from build123d import *

# Parameters (mm, degrees)
F0_W     = 5.842
F0_H     = 12.7
F0_R     = 3.175
F2_DEPTH = 25.4


with BuildPart() as f1:
    # F0 (on Front) → F1 (revolve)
    with BuildSketch(Plane.XZ):
        with Locations((2.921, 6.35)):
            Rectangle(F0_W, F0_H)
        Polygon((5.842, 12.7), (5.842, 0), (66.294, 0), (66.294, 12.7), (56.134, 12.7), (56.134, 10.16), (10.16, 10.16), (10.16, 12.7), align=None)
    revolve(axis=Axis((33.147, 0, 0), (-1, 0, 0)))

    # F0 (on Front) → F2 (join)
    with BuildSketch(Plane.XZ):
        with BuildLine():
            Line((-0.9398, 0), (0, 0))
            Line((0, 0), (0, 12.7))
            Line((0, 12.7), (5.842, 12.7))
            Line((5.842, 12.7), (5.842, 15.24))
            Line((5.842, 15.24), (-0.508, 15.24))
            Line((-0.508, 15.24), (-10.88063, 3.847543))
            ThreePointArc((-10.88063, 3.847543), (-4.591961, 5.329721), (-0.9398, 0))
        make_face()
        with BuildLine():
            ThreePointArc((-8.182663, -5.506983), (-3.195791, -4.549339), (-0.9398, 0))
            ThreePointArc((-0.9398, 0), (-4.591961, 5.329721), (-10.88063, 3.847543))
            ThreePointArc((-10.88063, 3.847543), (-12.145978, -1.583727), (-8.182663, -5.506983))
        make_face()
        with Locations((-6.6548, 0)):
            Circle(F0_R, mode=Mode.SUBTRACT)
        with BuildLine():
            Line((5.842, 0), (0, 0))
            Line((0, 0), (-0.9398, 0))
            ThreePointArc((-0.9398, 0), (-3.195791, -4.549339), (-8.182663, -5.506983))
            Line((-8.182663, -5.506983), (5.842, -9.398))
            Line((5.842, -9.398), (5.842, 0))
        make_face()
        with Locations((2.921, 6.35)):
            Rectangle(F0_W, F0_H)
    extrude(amount=F2_DEPTH)


solid = f1.part
Geometry: final body of the model. Coordinates: model frame, mm. A direction names the side the tool comes from. Round coordinates to 2 decimals unless told otherwise and drop trailing zeros. Loops run counter-clockwise (first coordinate to the right, second up) from the corner with the lowest first, then second, coordinate; pieces in that order, holes last.
Q1. Access query for faces 1 (the flat face through (-5.622, -12.522, 9.624)), 2 (the flat face through (10.16, 9, 6)), 3 (the cylindrical face through (61.14, -12.4, -2.75)), 4 (the flat face through (0, 4, -3)), 5 (the flat face through (-1.269, -15.344, -7.425)). Directions: +Z, -Z, +X, -X, +Y, -Y. A direction counts if a zero-diameter tool reaches every point of the face in a straight line with its end or side. Return the directions, or none.
Q2. Section C-C on y = 9. Return loops of the section in (x, z).
Q3. Pin query (flat end, axial travel): P1, Ø4, axis at x = 14, z = -0.5, coming from the +Y side; P2, Ø8, axis at x = 53.5, y = -5, coming from the +Z side; P3, Ø5.5, axis at x = -7, z = 1.5, coming from the +Y side. Return the tip coordinate at first contact, or that it passes through.
Q4. Section A-A on z = 0. Return loops of the section in (x, y).
Q5. Section B-B on y = -15. Return loops of the section in (x, z) (3 decimals), plus the area to 3 significant figures.
Q6. Section D-D on z = -11. Return loops of the section in (x, y).
Q7. Pull-direction query (Z, two-part tool) for faces 6 (the cylindrical face through (32.825, 10.074, -1.323)), 7 (the flat face through (-1, -25.4, 3)), 8 (the cylindrical face through (-3.626, -12.522, 0.954)), 9 (the flat face through (3, -13, 15.24)); classes: released by +Z, released by -Z, zero draft, split by the parting line, or undercut.
Q8. Material intervals for L1, parallel to X at y = -2, z = -10; L2, parallel to X at y = 5, z = -5.75; L3, parallel to Z at x = -8, y = -18.5, sorted ascending.
Evaluation:
1. face 1: +Z, -X, +Y, -Y
1. face 2: none
1. face 3: +X
1. face 4: -Z, -X, +Y
1. face 5: -Z, -X, -Y
2. outline: (0, -8.96) - (10.16, -8.96) - (10.16, -4.71) - (56.13, -4.71) - (56.13, -8.96) - (66.29, -8.96) - (66.29, 8.96) - (56.13, 8.96) - (56.13, 4.71) - (10.16, 4.71) - (10.16, 8.96) - (0, 8.96) - close
3. P1: stops at y = 10.16
3. P2: stops at z = 12.54
3. P3: stops at y = 0
4. outline: (-12.37, -25.4) - (-9.83, -25.4) - (-9.83, 0) - (-12.37, 0) - close; (-3.48, -25.4) - (5.84, -25.4) - (5.84, -12.7) - (10.16, -12.7) - (10.16, -10.16) - (56.13, -10.16) - (56.13, -12.7) - (66.29, -12.7) - (66.29, 12.7) - (56.13, 12.7) - (56.13, 10.16) - (10.16, 10.16) - (10.16, 12.7) - (0, 12.7) - (0, 0) - (-3.48, 0) - close
5. outline: (-10.881, 3.848) arc R5.715 ccw to (-8.183, -5.507) - (5.842, -9.398) - (5.842, 15.24) - (-0.508, 15.24) - close; hole circle Ø6.35 at (-6.655, 0)
5. area: 290 mm2
6. outline: (0, -6.35) - (10.16, -6.35) - (10.16, 6.35) - (0, 6.35) - close; (56.13, -6.35) - (66.29, -6.35) - (66.29, 6.35) - (56.13, 6.35) - close
7. face 6: split by the parting line
7. face 7: zero draft
7. face 8: undercut
7. face 9: released by +Z
8. L1: x = 0 to 10.16, 56.13 to 66.29
8. L2: x = 0 to 66.29
8. L3: z = -5.56 to -2.88, 2.88 to 7.01
